CAD build for the part. Positions are in the model's coordinates, mm. Give positions to 0.01 mm unless a question says otherwise; leave off trailing zeros. Order: outer loops, then holes, each group sorted by start corner. A loop starts at its lowest first (then second) coordinate and runs counter-clockwise, first axis right, second up. Notation, with made-up numbers: M -25.75,26.25 L 14.25,26.25 A20 ccw 14.25,40.25 Z; hole C 87.5,19.25 d8. An arc over 180 degrees is marked long. Put each result on its own line as item: value. Start each with the question number.
1) Drill centre lines: line 1 (X direction, y = -12.75, z = 56); line 2 (Z direction, x = 37, y = -22.5); line 3 (X direction, y = -2.25, z = 33). Where is each one in solid material? Low to high. Write a range as [from, to].
2) Cut at B-B (x = 22). Write the cut outline in (y, z).
3) Pin check, flat tips, straight feed: pin 1 (3 mm diameter, centred on x = -13, y = -20, fed in from +Z); pin 2 (8 mm diameter, centred on x = -39, z = 48.5, fed in from -Y) (1 decimal); pin 3 (4 mm diameter, centred on x = 29.5, y = -18, fed in from +Z); pin 4 (5 mm diameter, centred on x = -3.5, y = -8, fed in from +Z). Stop position of each tip, or through.
4) Cut at C-C (z = 42.5). Write the cut outline in (x, y), and give its area (3 significant figures).
5) Cut at A-A (y = -5). Write the cut outline in (x, z).
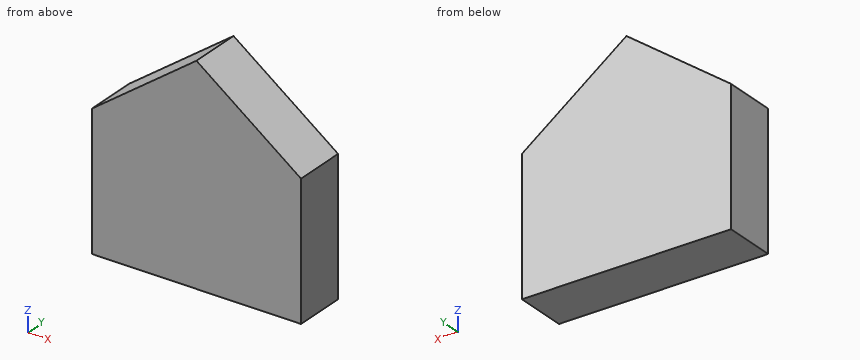
```python
from build123d import *

# Parameters (mm, degrees)
F0_W     = 101.417362
F0_H     = 65.29244
F1_DEPTH = 25.4


with BuildPart() as f1:
    # F0 (on Front) → F1 (new body)
    with BuildSketch(Plane.XZ):
        Rectangle(F0_W, F0_H)
        Polygon((-50.708681, 32.64622), (50.708681, 32.64622), (0, 69.841512), align=None)
    extrude(amount=F1_DEPTH)


solid = f1.part
```
Solution:
1. line 1: [-18.87, 18.87]
1. line 2: [-32.65, 42.7]
1. line 3: [-50.23, 50.23]
2. outline: M -25.4,-32.65 L 0,-32.65 L 0,53.7 L -25.4,53.7 Z
3. pin 1: z = 61.41
3. pin 2: through
3. pin 3: z = 49.67
3. pin 4: z = 69.11
4. outline: M -37.27,-25.4 L 37.27,-25.4 L 37.27,0 L -37.27,0 Z
4. area: 1,890 mm²
5. outline: M -50.71,-32.65 L 50.71,-32.65 L 50.71,32.65 L 0,69.84 L -50.71,32.65 Z
